Could you check a few things on this drawing? It's one solid part, dimensions in mm from its lowest x, y, z. Coordinates: 2 decimals unless noted, no trailing zeros. Loops run counter-clockwise (first coordinate to the right, second up) from the corner with the lowest first, then second, coordinate; pieces in that order, holes last. Notation, with made-up numbers: M -33,18 L -23,18 A14 ccw -23,31 Z; hole C 35.5,18 d1. An arc over 180 degrees is marked long. Answer as a JSON object with one key per item and string values. Group by question number.
Item 1: We'd pull the mould along X, two halves only. Please class the marked faces 1 and 2: +X half, -X half, draft (parallel to the pull), parting line (faces both ways), or undercut.
Item 2: If I drill on line 1 (Y direction, x = 63.5, z = 8.25); line 2 (Y direction, x = 31.5, z = 4.5); line 3 (X direction, y = 57, z = 9.5), over which ranges is the centre line in solid material (lowest first)?
Item 3: Suppose I cut it at C-C (z = 5.25). Write out the boundary of the cut face in (x, y), then the cut area to 3 significant figures.
Item 4: Suppose I cut it at A-A (y = 63.5). Write out the boundary of the cut face in (x, z), then the cut area to 3 significant figures.
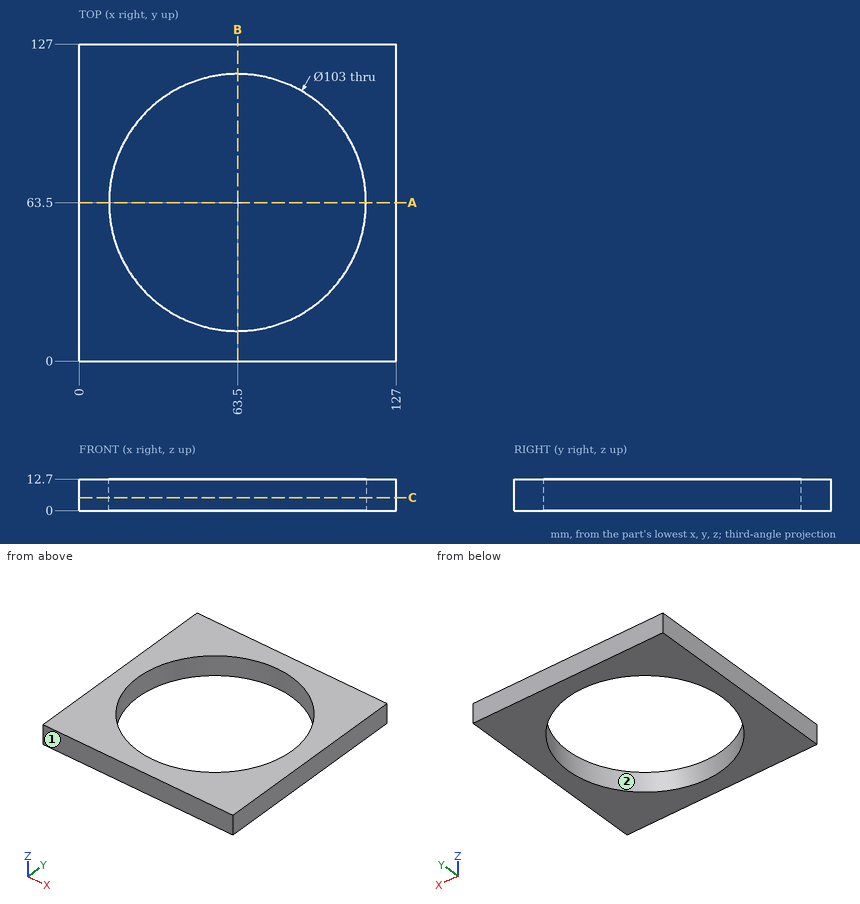
From the geometry:
{
 "1": {"face 1": "draft", "face 2": "undercut"},
 "2": {"line 1": "0 to 12, 115 to 127", "line 2": "0 to 23.15, 103.85 to 127", "line 3": "0 to 12.41, 114.59 to 127"},
 "3": {"outline": "M 0,0 L 127,0 L 127,127 L 0,127 Z; hole C 63.5,63.5 d103", "area": "7,800 mm2"},
 "4": {"outline": "M 0,0 L 12,0 L 12,12.7 L 0,12.7 Z; M 115,0 L 127,0 L 127,12.7 L 115,12.7 Z", "area": "305 mm2"}
}
